Can you work these out from the drawing? Everything is in mm from the part's minimum corner. Round coordinates to 2 decimals unless told otherwise and drop trailing zeros. Write each loop counter-clockwise with the first axis right and the second up, starting at its lowest first coordinate (ties: lowest second). Pieces come first, ordered by that corner, then holes. Notation, with made-up numbers: (45, 13) - (62, 13) arc R27 ccw to (62, 47) - close; hole circle Ø9 at (-9.75, 82.5). An arc over 180 degrees is marked (long way). One line per item, written item: value. Start each with the question number.
Item 1: Imagine slicing it at C-C, the plane z = 0.6. Please give me the cut outline in (x, y), then the cut area to 3 significant figures.
Item 2: If I drill on line 1 (X direction, y = 3.5, z = 0.6); line 2 (Y direction, x = 7, z = 1.05); line 3 (Y direction, x = 7, z = 0.8), over which ranges is the centre line in solid material (lowest first)?
Item 3: Imagine slicing it at D-D, the plane x = 10.75. Please give me the cut outline in (y, z).
Item 4: Imagine slicing it at A-A, the plane x = 7. Please give me the cut outline in (y, z).
Item 5: Thinking about a two-plate mould opening in X: for the marked faces 1, 2, 3 and 4, which applies, released by +X, released by -X, zero draft, split by the parting line, or undercut?
Item 6: For P1, Ø1, axis at y = 8, z = 1, coming from the +X side, with a flat end and sliding along its axis, tell me the tip position at first contact or that it passes through.
Item 7: Imagine slicing it at B-B, the plane y = 3.5. Please give me the cut outline in (x, z).
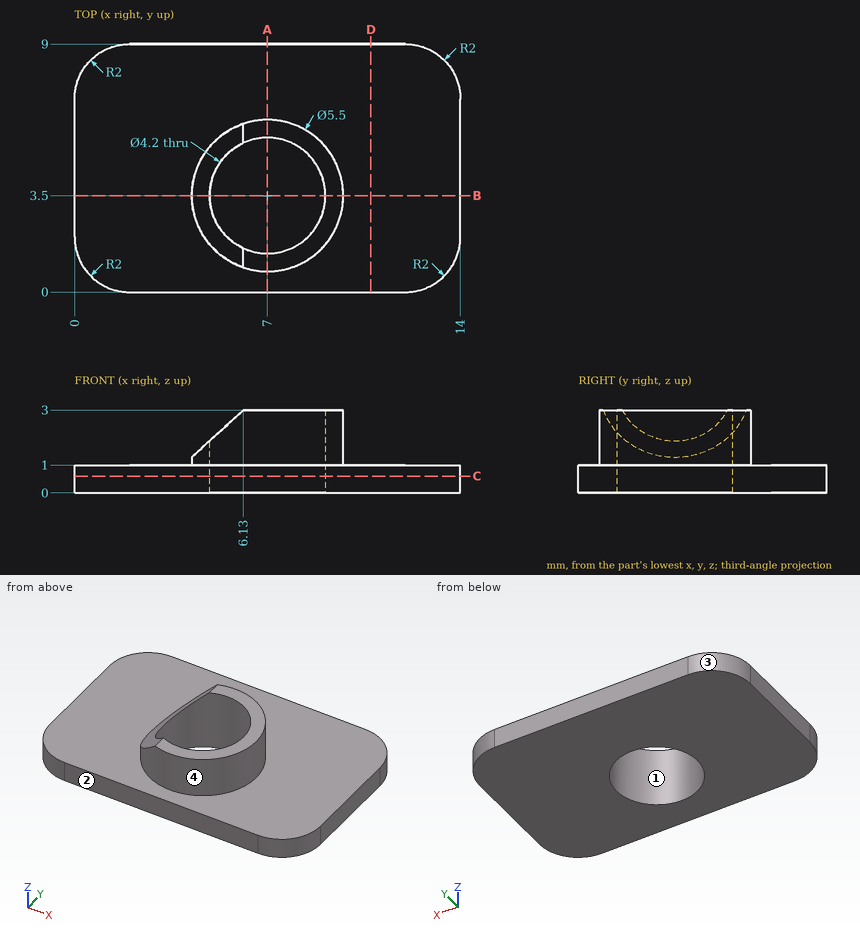
Values follow:
1. outline: (0, 2) arc R2 ccw to (2, 0) - (12, 0) arc R2 ccw to (14, 2) - (14, 7) arc R2 ccw to (12, 9) - (2, 9) arc R2 ccw to (0, 7) - close; hole circle Ø4.2 at (7, 3.5)
1. area: 109 mm^2
2. line 1: x = 0 to 4.9, 9.1 to 14
2. line 2: y = 0.75 to 1.4, 5.6 to 6.25
2. line 3: y = 0 to 1.4, 5.6 to 9
3. outline: (0, 0) - (9, 0) - (9, 1) - (0, 1) - close
4. outline: (0, 0) - (1.4, 0) - (1.4, 3) - (0.75, 3) - (0.75, 1) - (0, 1) - close; (5.6, 0) - (9, 0) - (9, 1) - (6.25, 1) - (6.25, 3) - (5.6, 3) - close
5. face 1: undercut
5. face 2: zero draft
5. face 3: released by -X
5. face 4: split by the parting line
6. P1: stops at x = 13.94
7. outline: (0, 0) - (4.9, 0) - (4.9, 1.88) - (4.25, 1.29) - (4.25, 1) - (0, 1) - close; (9.1, 0) - (14, 0) - (14, 1) - (9.75, 1) - (9.75, 3) - (9.1, 3) - close
